from build123d import *

# Parameters (mm, degrees)
MAINBLOCKSKETCH_W              = 26.5
MAINBLOCKSKETCH_H              = 45.4
MAINBLOCK_DEPTH                = 9
FACEDSURFACESKETCH_W           = 27
FACEDSURFACESKETCH_H           = 32.4
FACEDSURFACE_DEPTH             = 10
M3X0_5_TAPPED_HOLE1_D          = 2.5
M3X0_5_TAPPED_HOLE1_DEPTH      = 8.5
M3X0_5_TAPPED_HOLE1_TIP        = 0.751075774
RAIL_SLOT_DEPTH                = 29.240750698
RAIL_SLOT_DEPTH_BACK           = 29.240750698
INTERNAL_DIP_SKETCH_W          = 13.5
INTERNAL_DIP_SKETCH_H          = 32.4
INTERNAL_DIP_DEPTH             = 0.9
INTERNAL_CHAMFER_SIZE          = 0.5
COSMETIC_CHAMFERS_SIZE         = 1
SMALLER_COSMETIC_CHAMFERS_SIZE = 0.5


with BuildPart() as part:
    # MainBlockSketch → MainBlock (new body)
    with BuildSketch(Plane(origin=(0, 0, 0), x_dir=(1, 0, 0), z_dir=(0, 1, 0))):
        Rectangle(MAINBLOCKSKETCH_W, MAINBLOCKSKETCH_H)
    extrude(amount=MAINBLOCK_DEPTH)

    # FacedSurfaceSketch → FacedSurface (add)
    with BuildSketch(Plane(origin=(0, 0, 0), x_dir=(1, 0, 0), z_dir=(0, 1, 0))):
        Rectangle(FACEDSURFACESKETCH_W, FACEDSURFACESKETCH_H)
    extrude(amount=FACEDSURFACE_DEPTH)

    # M3x0.5 Tapped Hole1
    with Locations(Plane(origin=(0, 10, 0), x_dir=(1, 0, 0), z_dir=(0, 1, 0))):
        with Locations((-10, 10), (10, 10), (10, -10), (-10, -10)):
            Hole(M3X0_5_TAPPED_HOLE1_D / 2, depth=M3X0_5_TAPPED_HOLE1_DEPTH)
            with Locations((0, 0, -(M3X0_5_TAPPED_HOLE1_DEPTH + M3X0_5_TAPPED_HOLE1_TIP / 2))):  # 118° drill point
                Cone(0, M3X0_5_TAPPED_HOLE1_D / 2, M3X0_5_TAPPED_HOLE1_TIP, mode=Mode.SUBTRACT)

    # RailSlotSketch → Rail Slot (cut, two sides: drawn at the far end of the back side and taken through both)
    with BuildSketch(Plane.XY.offset(-RAIL_SLOT_DEPTH_BACK)):
        with BuildLine():
            Line((-6, 2.59), (-6, 5))
            Line((-6, 5), (6, 5))
            Line((6, 5), (6, 2.59))
            ThreePointArc((6, 2.59), (5.2, 1.79), (6, 0.99))
            Line((6, 0.99), (6, 0))
            Line((6, 0), (-6, 0))
            Line((-6, 0), (-6, 0.99))
            ThreePointArc((-6, 0.99), (-5.2, 1.79), (-6, 2.59))
        make_face()
    extrude(amount=RAIL_SLOT_DEPTH + RAIL_SLOT_DEPTH_BACK, mode=Mode.SUBTRACT)

    # Internal Dip Sketch → Internal Dip (cut)
    with BuildSketch(Plane(origin=(0, 10, 0), x_dir=(1, 0, 0), z_dir=(0, 1, 0))):
        Rectangle(INTERNAL_DIP_SKETCH_W, INTERNAL_DIP_SKETCH_H)
    extrude(amount=-INTERNAL_DIP_DEPTH, mode=Mode.SUBTRACT)

    # Internal Chamfer
    internal_chamfer_edges = [part.edges().sort_by_distance(p)[0] for p in [
        (6, 5, 0),
        (-6, 5, 0),
    ]]
    chamfer(internal_chamfer_edges, length=INTERNAL_CHAMFER_SIZE)

    # Cosmetic Chamfers
    # the kernel refuses this chamfer: 1 mm, written as the material it adds along each edge
    with BuildSketch(Plane(origin=(-6.75, 9.1, 16.2), x_dir=(0.9996219169112968, -0.027495876610585623, 0), z_dir=(0, 0, -1))) as cosmetic_chamfers_piece_1_section:
        Polygon((COSMETIC_CHAMFERS_SIZE * 0.999621916911, -COSMETIC_CHAMFERS_SIZE * 0.0274958766106), (-COSMETIC_CHAMFERS_SIZE * 0.0274958766106, -COSMETIC_CHAMFERS_SIZE * 0.999621916911), (0, 0), align=None)
    cosmetic_chamfers_piece_1 = extrude(amount=32.4, mode=Mode.PRIVATE)
    cosmetic_chamfers_piece_1 = split(cosmetic_chamfers_piece_1, bisect_by=Plane(origin=(-6.414099253, 10, 0), z_dir=(0, -1, 0)), keep=Keep.TOP, mode=Mode.PRIVATE)
    add(cosmetic_chamfers_piece_1)
    with BuildSketch(Plane(origin=(6.75, 9.1, -16.2), x_dir=(0.02749587661058651, 0.9996219169112968, 0), z_dir=(0, 0, 1))) as cosmetic_chamfers_piece_2_section:
        Polygon((COSMETIC_CHAMFERS_SIZE * 0.999621916911, COSMETIC_CHAMFERS_SIZE * 0.0274958766106), (-COSMETIC_CHAMFERS_SIZE * 0.0274958766106, COSMETIC_CHAMFERS_SIZE * 0.999621916911), (0, 0), align=None)
    cosmetic_chamfers_piece_2 = extrude(amount=32.4, mode=Mode.PRIVATE)
    cosmetic_chamfers_piece_2 = split(cosmetic_chamfers_piece_2, bisect_by=Plane(origin=(6.414099253, 10, 0), z_dir=(0, -1, 0)), keep=Keep.TOP, mode=Mode.PRIVATE)
    add(cosmetic_chamfers_piece_2)
    # the kernel refuses this chamfer: 1 mm, written as the material it takes off along each edge
    with BuildSketch(Plane(origin=(13.25, 9, 25.271682988), x_dir=(0.027495876610585623, -0.9996219169112968, 0), z_dir=(0, 0, -1))) as cosmetic_chamfers_2_piece_1:
        Polygon((COSMETIC_CHAMFERS_SIZE * 0.999621916911, COSMETIC_CHAMFERS_SIZE * 0.0274958766106), (-COSMETIC_CHAMFERS_SIZE * 0.0274958766106, COSMETIC_CHAMFERS_SIZE * 0.999621916911), (0, 0), align=None)
    extrude(amount=9.071682988, mode=Mode.SUBTRACT)
    with BuildSketch(Plane(origin=(-13.25, 9, 16.2), x_dir=(0.9996219169112968, 0.027495876610585647, 0), z_dir=(0, 0, 1)), Plane(origin=(-13.25, 9, -25.271682988), x_dir=(0.9996219169112968, 0.027495876610585647, 0), z_dir=(0, 0, 1)), Plane(origin=(13.25, 9, -16.2), x_dir=(-0.9996219169112968, 0.027495876610585647, 0), z_dir=(0, 0, -1))) as cosmetic_chamfers_2_piece_2:
        Polygon((COSMETIC_CHAMFERS_SIZE * 0.999621916911, -COSMETIC_CHAMFERS_SIZE * 0.0274958766106), (-COSMETIC_CHAMFERS_SIZE * 0.0274958766106, -COSMETIC_CHAMFERS_SIZE * 0.999621916911), (0, 0), align=None)
    extrude(amount=9.071682988, mode=Mode.SUBTRACT)

    # Smaller Cosmetic Chamfers
    smaller_cosmetic_chamfers_edges = [part.edges().sort_by_distance(p)[0] for p in [
        (13.5, 10, 0),
        (-13.5, 10, 0),
        (-13.5, 0, 0),
        (13.5, 0, 0),
        (6, 0, 0),
        (-6, 0, 0),
    ]]
    chamfer(smaller_cosmetic_chamfers_edges, length=SMALLER_COSMETIC_CHAMFERS_SIZE)


solid = part.part
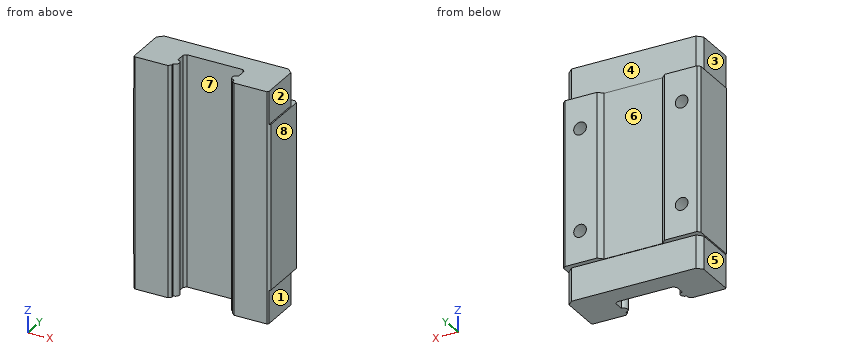
The listing builds one solid part. Answer for the finished solid, in the listing's coordinates (mm). Face numbers are marked on the shaded views. A direction names the side the tool comes from. Round coordinates to 2 decimals unless told otherwise and drop trailing zeros. Loops run counter-clockwise (first coordinate to the right, second up) from the corner with the lowest first, then second, coordinate; pieces in that order, holes last. Notation, with made-up numbers: M 35,10 L 91,10 A12 cw 91,19 Z; hole C 87.5,-22 d9. An arc over 180 degrees is marked long. Return JSON: item names as keys, results as strings.
Q1. The mould has two halves that part along X. Classify the marked faces 5, 6, 7 and 8: released by +X, released by -X, zero draft, split by the parting line, or undercut.
Results list:
{"face 5": "released by -X", "face 6": "undercut", "face 7": "undercut", "face 8": "released by +X"}
Q2. Find section C-C, the plane x = -2.5. Determine the outline of the cut face in (y, z).
Results list:
{"outline": "M 5,-22.7 L 9,-22.7 L 9,-16.2 L 9.1,-16.2 L 9.1,16.2 L 9,16.2 L 9,22.7 L 5,22.7 Z"}
Q3. Find the intervals of material crossed by line 1 along X through (y, z) = (6.5, 10); line 2 along Z through (x, y) = (10, 3.5); line 3 along X through (y, z) = (4.5, 10), in increasing order. Write a range as from..to.
Results list:
{"line 1": "x = -13.5..-11.25, -8.75..8.75, 11.25..13.5", "line 2": "z = -22.7..-11.25, -8.75..8.75, 11.25..22.7", "line 3": "x = -13.5..-11.25, -8.75..-6, 6..8.75, 11.25..13.5"}
Q4. Which of the six approach directions +Z, -Z, +X, -X, +Y, -Y give full straight-line access (tool end or side, diameter ignored) to the marked faces 1, 2, 3 and 4?
Results list:
{"face 1": "-Z, +X, +Y, -Y", "face 2": "+Z, +X, +Y, -Y", "face 3": "+Z, -X, +Y, -Y", "face 4": "+Z, +X, -X, +Y"}
Q5. Find section D-D, the plane z = -4. Determine the outline of the cut face in (x, y).
Results list:
{"outline": "M -13.5,0.5 L -13,0 L -6.5,0 L -6,0.5 L -6,0.99 A0.8 ccw -6,2.59 L -6,4.5 L -5.5,5 L 5.5,5 L 6,4.5 L 6,2.59 A0.8 ccw 6,0.99 L 6,0.5 L 6.5,0 L 13,0 L 13.5,0.5 L 13.5,9.5 L 13,10 L 6.65,10 L 5.75,9.1 L -5.75,9.1 L -6.65,10 L -13,10 L -13.5,9.5 Z"}
Q6. Find section A-A, the plane y = 2. Determine the outline of the cut face in (x, z), plus the area to 3 significant figures.
Results list:
{"outline": "M -13.5,-16.2 L -13.25,-16.2 L -13.25,-22.7 L -5.23,-22.7 L -5.23,22.7 L -13.25,22.7 L -13.25,16.2 L -13.5,16.2 Z; M 5.23,-22.7 L 13.25,-22.7 L 13.25,-16.2 L 13.5,-16.2 L 13.5,16.2 L 13.25,16.2 L 13.25,22.7 L 5.23,22.7 Z; hole C -10,-10 d2.5; hole C -10,10 d2.5; hole C 10,-10 d2.5; hole C 10,10 d2.5", "area": "725 mm2"}
Q7. Find section B-B, the plane z = -17. Determine the outline of the cut face in (x, y), plus the area to 3 significant figures.
Results list:
{"outline": "M -13.25,0.25 L -13,0 L -6.5,0 L -6,0.5 L -6,0.99 A0.8 ccw -6,2.59 L -6,4.5 L -5.5,5 L 5.5,5 L 6,4.5 L 6,2.59 A0.8 ccw 6,0.99 L 6,0.5 L 6.5,0 L 13,0 L 13.25,0.25 L 13.25,8 L 12.25,9 L -12.25,9 L -13.25,8 Z", "area": "179 mm2"}
Q8. Each of these flat-tipped pins is pushed along its axis until it touches: pin 1 Ø3 at (x, z) = (2.5, -21) entering from +Y; pin 2 Ø5 at (y, z) = (2.5, -20) entering from +X; pin 3 Ø3 at (x, z) = (-10, -10) entering from +Y. Where does it stop, or does it pass through?
Results list:
{"pin 1": "stops at y = 9", "pin 2": "stops at x = 13.25", "pin 3": "stops at y = 10"}
